CAD build for the part. Positions are in the model's coordinates, mm. Face numbers are marked on the shaded views. A direction names the side the tool comes from. Give positions to 0.01 mm unless a question says otherwise; leave off trailing zeros. Loops run counter-clockwise (first coordinate to the right, second up) from the corner with the lowest first, then second, coordinate; pieces in that order, holes last. Notation, with made-up numbers: M 75.5,6.25 L 82.5,6.25 A17 cw 82.5,25.25 Z; hole C 25,-39 d1. An arc over 180 degrees is marked long. Answer as CSV lines item,"result".
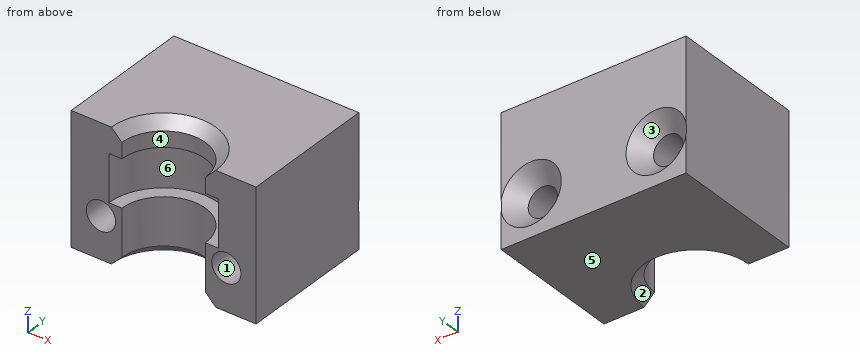
```python
from build123d import *

# Parameters (mm, degrees)
SKETCH_2_W            = 17.7
SKETCH_2_H            = 13
EXTRUDE_380_DEPTH     = 6.25
SKETCH_3_R            = 4
CUT_EXTRUDE_527_DEPTH = 21.089113968
CUT_EXTRUDE_START     = -2.5
SKETCH_4_R            = 5.25
CUT_EXTRUDE_676_DEPTH = 4.5
SKETCH_5_R            = 1.4
CUT_EXTRUDE_872_DEPTH = 17.922913461
CHAMFER_2_SIZE        = 1
CHAMFER_3_SIZE        = 1.5


with BuildPart() as part:
    # Эскиз2 → Extrude 380 (new, symmetric)
    with BuildSketch(Plane.XY):
        with Locations((0, 6.5)):
            Rectangle(SKETCH_2_W, SKETCH_2_H)
    extrude(amount=EXTRUDE_380_DEPTH, both=True)

    # Эскиз3 → Cut-Extrude 527 (cut, through all)
    with BuildSketch(Plane.XY.offset(6.25)):
        Circle(SKETCH_3_R)
    extrude(amount=-CUT_EXTRUDE_527_DEPTH, mode=Mode.SUBTRACT)

    # Эскиз4 → Cut-Extrude 676 (cut)
    with BuildSketch(Plane.XY.offset(6.25).offset(CUT_EXTRUDE_START)):
        Circle(SKETCH_4_R)
    extrude(amount=-CUT_EXTRUDE_676_DEPTH, mode=Mode.SUBTRACT)

    # Эскиз5 → Cut-Extrude 872 (cut, through all)
    with BuildSketch(Plane(origin=(0, 13, 0), x_dir=(1, 0, 0), z_dir=(0, 1, 0))):
        with Locations(Location((-6, 2.25, 0), (0, 0, 270))):
            Circle(SKETCH_5_R)
        with Locations(Location((6, 2.25, 0), (0, 0, 270))):
            Circle(SKETCH_5_R)
    extrude(amount=-CUT_EXTRUDE_872_DEPTH, mode=Mode.SUBTRACT)

    # Фаска2
    chamfer_2_edges = [part.edges().sort_by_distance(p)[0] for p in [
        (0, 4, 6.25),
        (0, 4, -6.25),
    ]]
    chamfer(chamfer_2_edges, length=CHAMFER_2_SIZE)

    # Фаска3
    # the kernel refuses this chamfer: 1.5 mm, written as the material it takes off along each edge
    with BuildSketch(Plane(origin=(-6, 13, -2.25), x_dir=(0, 0, 1), z_dir=(-1, 0, 0))) as chamfer_3_piece_1:
        Polygon((1.4 + CHAMFER_3_SIZE, 0), (1.4, -CHAMFER_3_SIZE), (1.4, 0), align=None)
    revolve(axis=Axis((-6, 13, -2.25), (0, 1, 0)), mode=Mode.SUBTRACT)
    with BuildSketch(Plane(origin=(6, 13, -2.25), x_dir=(0, 0, 1), z_dir=(-1, 0, 0))) as chamfer_3_piece_2:
        Polygon((1.4, -CHAMFER_3_SIZE), (1.4 + CHAMFER_3_SIZE, 0), (1.4, 0), align=None)
    revolve(axis=Axis((6, 13, -2.25), (0, 1, 0)), mode=Mode.SUBTRACT)


solid = part.part
```
Q1. Which spindle directions (+Z, -Z, +X, -X, +Y, -Y) get a long thin tool onto all of the face, cutting with end or side? Do the marked faces 5 and 6. Say none if no direction does.
Solution:
face 5,"-Z, +X, -X, +Y, -Y"
face 6,"-Y"
Q2. Cut at C-C (x = 0). Write the cut outline in (y, z), and give its area (3 significant figures).
Solution:
outline,"M 4,-5.25 L 5,-6.25 L 13,-6.25 L 13,6.25 L 5,6.25 L 4,5.25 L 4,3.75 L 5.25,3.75 L 5.25,-0.75 L 4,-0.75 Z"
area,"106 mm²"
Q3. Cut at A-A (x = 6). Write the cut outline in (y, z), and give its area (3 significant figures).
Solution:
outline,"M 0,-6.25 L 13,-6.25 L 13,-5.15 L 11.5,-3.65 L 0,-3.65 Z; M 0,-0.85 L 11.5,-0.85 L 13,0.65 L 13,6.25 L 0,6.25 Z"
area,"124 mm²"
Q4. Cut at D-D (y = 2.25). Give the number of separate pieces and of enclosed holes in the cut face, and give its area (3 significant figures).
Solution:
separate pieces,"2"
enclosed holes,"2"
area,"111 mm²"
Q5. Cut at B-B (y = 11). Write the cut outline in (x, z).
Solution:
outline,"M -8.85,-6.25 L 8.85,-6.25 L 8.85,6.25 L -8.85,6.25 Z; hole C -6,-2.25 d2.8; hole C 6,-2.25 d2.8"
Q6. Wall check: line 1 (X direction, y = 6, z = -2.25); line 2 (X direction, y = 3.25, z = -2.25); line 3 (X direction, y = 5.25, z = -2.75). Give the ranges that are in metal, low to high. Write a range as [from, to].
Solution:
line 1,"x = [-8.85, -7.4], [-4.6, 4.6], [7.4, 8.85]"
line 2,"x = [-8.85, -7.4], [-4.6, -2.33], [2.33, 4.6], [7.4, 8.85]"
line 3,"x = [-8.85, -7.31], [-4.69, 4.69], [7.31, 8.85]"
Q7. Mould opens along Z. For the marked faces 1, 2, 3 and 4 say: released by +Z, released by -Z, zero draft, split by the parting line, or undercut.
Solution:
face 1,"undercut"
face 2,"released by -Z"
face 3,"undercut"
face 4,"zero draft"
